```python
from build123d import *

# Parameters (mm, degrees)
SKETCH_1_R      = 10
SKETCH_1_R_2    = 7.55
SKETCH_1_R_3    = 1.65
SKETCH_1_R_4    = 1.6
EXTRUDE_1_DEPTH = 5


with BuildPart() as part:
    # 草图1 → 凸台-拉伸1 (new body)
    with BuildSketch(Plane(origin=(0, 0, 0), x_dir=(1, 0, 0), z_dir=(0, 1, 0))):
        with BuildLine():
            Line((-35, 33), (35, 33))
            ThreePointArc((35, 33), (38.535533906, 31.535533906), (40, 28))
            Line((40, 28), (40, -15))
            ThreePointArc((40, -15), (38.535533906, -18.535533906), (35, -20))
            Line((35, -20), (-35, -20))
            ThreePointArc((-35, -20), (-38.535533906, -18.535533906), (-40, -15))
            Line((-40, -15), (-40, 28))
            ThreePointArc((-40, 28), (-38.535533906, 31.535533906), (-35, 33))
        make_face()
        Circle(SKETCH_1_R, mode=Mode.SUBTRACT)
        with Locations((-25, 0)):
            Circle(SKETCH_1_R_2, mode=Mode.SUBTRACT)
        with Locations((-33.485281374, 8.485281374)):
            Circle(SKETCH_1_R_3, mode=Mode.SUBTRACT)
        with Locations((-16.514718626, 8.485281374)):
            Circle(SKETCH_1_R_3, mode=Mode.SUBTRACT)
        with Locations((-16.514718626, -8.485281374)):
            Circle(SKETCH_1_R_3, mode=Mode.SUBTRACT)
        with Locations((-33.485281374, -8.485281374)):
            Circle(SKETCH_1_R_3, mode=Mode.SUBTRACT)
        with Locations((25, 0)):
            Circle(SKETCH_1_R_2, mode=Mode.SUBTRACT)
        with Locations((16.514718626, 8.485281374)):
            Circle(SKETCH_1_R_3, mode=Mode.SUBTRACT)
        with Locations((16.514718626, -8.485281374)):
            Circle(SKETCH_1_R_3, mode=Mode.SUBTRACT)
        with Locations((33.485281374, -8.485281374)):
            Circle(SKETCH_1_R_3, mode=Mode.SUBTRACT)
        with Locations((33.485281374, 8.485281374)):
            Circle(SKETCH_1_R_3, mode=Mode.SUBTRACT)
        with Locations((-20, 23)):
            Circle(SKETCH_1_R_4, mode=Mode.SUBTRACT)
        with Locations((0, 23)):
            Circle(SKETCH_1_R_4, mode=Mode.SUBTRACT)
        with Locations((20, 23)):
            Circle(SKETCH_1_R_4, mode=Mode.SUBTRACT)
    extrude(amount=EXTRUDE_1_DEPTH)


solid = part.part
```
Could you check a few things on this model? Use its own coordinates, in mm. Give positions to 0.01 mm unless a question says otherwise; leave off trailing zeros. Order: outer loops, then holes, each group sorted by start corner. A loop starts at its lowest first (then second) coordinate and runs counter-clockwise, first axis right, second up.
Q1. Suppose I cut it at D-D, the plane y = 3.15. Count the separate pieces of the cut face and the enclosed holes in it, and give its area (3 significant figures).
Q2. We'd pull the mould along Z, two halves only. Please class faces 1 (the cylindrical face through (-38, 2, 19)), 2 (the cylindrical face through (18.82, 2.46, -24.08)), 3 (the flat face through (40, 2, -7)): +Z half, -Z half, draft (parallel to the pull), parting line (faces both ways), or undercut.
Q3. Suppose I cut it at C-C, the plane x = -25. Write out the boundary of the cut face in (y, z).
Q4. If I drill on line 1 along Z through (x, y) = (0, 1.75); line 2 along X through (y, z) = (3.4, -23); line 3 along X through (y, z) = (0.65, 0.5), over which ranges is the centre line in solid material (lowest first)?
Q5. Suppose I cut it at A-A, the plane z = 0. Write out the boundary of the cut face in (x, y).
Q6. Suppose I cut it at B-B, the plane x = 0. Write out the boundary of the cut face in (y, z), and give its area (3 significant figures).
Q7. I'm going to push a flat-ended pin straight in: P1, Ø2, axis at x = -16.51, z = -8.49, coming from the -Y side. Where does the tip first touch, or does it pass through?
Solution:
1. separate pieces: 1
1. enclosed holes: 14
1. area: 3,450 mm2
2. face 1: +Z half
2. face 2: undercut
2. face 3: draft
3. outline: (0, -33) - (5, -33) - (5, -7.55) - (0, -7.55) - close; (0, 7.55) - (5, 7.55) - (5, 20) - (0, 20) - close
4. line 1: z = -33 to -24.6, -21.4 to -10, 10 to 20
4. line 2: x = -40 to -21.6, -18.4 to -1.6, 1.6 to 18.4, 21.6 to 40
4. line 3: x = -40 to -32.53, -17.47 to -9.99, 9.99 to 17.47, 32.53 to 40
5. outline: (-40, 0) - (-32.55, 0) - (-32.55, 5) - (-40, 5) - close; (-17.45, 0) - (-10, 0) - (-10, 5) - (-17.45, 5) - close; (10, 0) - (17.45, 0) - (17.45, 5) - (10, 5) - close; (32.55, 0) - (40, 0) - (40, 5) - (32.55, 5) - close
6. outline: (0, -33) - (5, -33) - (5, -24.6) - (0, -24.6) - close; (0, -21.4) - (5, -21.4) - (5, -10) - (0, -10) - close; (0, 10) - (5, 10) - (5, 20) - (0, 20) - close
6. area: 149 mm2
7. P1: passes through
